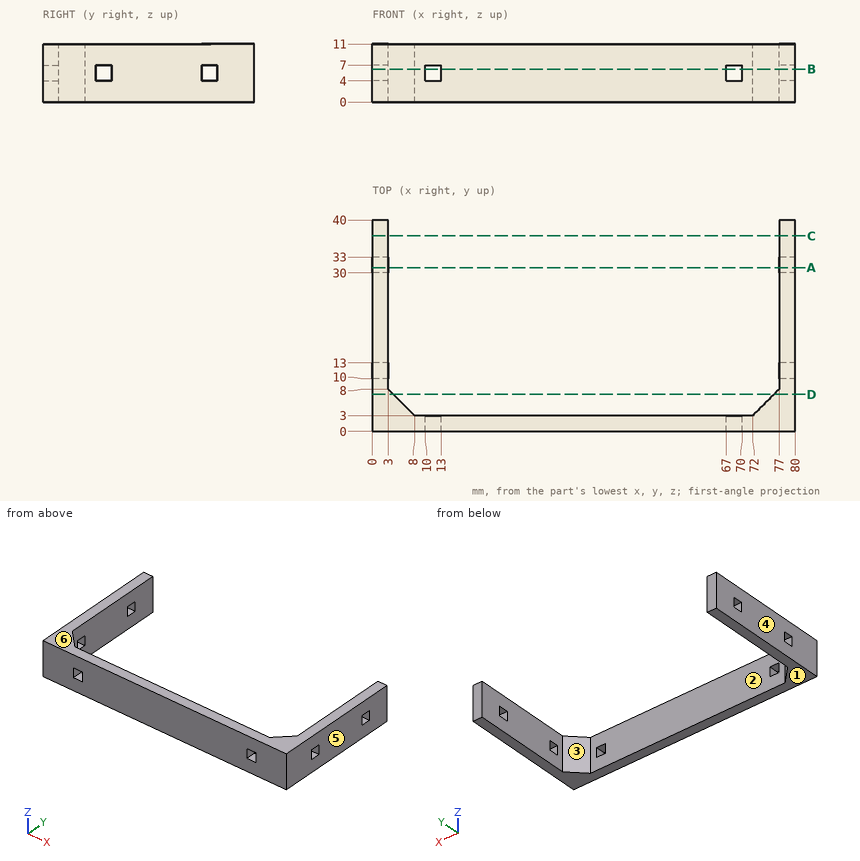
Job drawing, mm, ordinate dimensions from the low corner. One solid piece. A direction names the side the tool comes from. Coordinates: 2 decimals unless noted, no trailing zeros. Order: outer loops, then holes, each group sorted by start corner. A loop starts at its lowest first (then second) coordinate and runs counter-clockwise, first axis right, second up. Notation, with made-up numbers: (6, -3) - (10, -3) arc R36 ccw to (10, 33) - close; hole circle Ø5 at (66, 22.5). An arc over 180 degrees is marked (long way). Return JSON: item names as keys, results as strings. Group by question number.
1) Tool access for the marked faces 1 and 2: list every direction of +Z, -Z, +X, -X, +Y, -Y with a clear straight run to the whole face (end or side of a thin tool).
2) Probe line 1 (X direction, y = 2, z = 6.75); line 2 (X direction, y = 14, z = 9); line 3 (Y direction, x = 73, z = 9.75). List the from-to ranges inside material, lowest first. Write a range as from..to.
3) Mould opens along X. For the marked faces 3, 4, 5 and 6 say: released by +X, released by -X, zero draft, split by the parting line, or undercut.
4) Saw through at A-A, the plane y = 31. Write the cut outline in (x, z).
5) Saw through at C-C, the plane y = 37. Write the cut outline in (x, z), plus the area to 3 significant figures.
6) Saw through at D-D, the plane y = 7. Write the cut outline in (x, z).
7) Saw through at B-B, the plane z = 6.25. Count the separate pieces of the cut face and the enclosed holes in it, plus the area to 3 significant figures.
8) Flat gauge pin, fed straight in: P1, Ø2.5, axis at y = 1, z = 5, coming from the -X side. Where does the tip first touch, or does it go through?
Values found:
{
 "1": {"face 1": "-Z, +X, -X, +Y, -Y", "face 2": "+Z, -Z, +Y"},
 "2": {"line 1": "x = 0..10, 13..67, 70..80", "line 2": "x = 0..3, 77..80", "line 3": "y = 0..4"},
 "3": {"face 3": "undercut", "face 4": "released by -X", "face 5": "released by +X", "face 6": "zero draft"},
 "4": {"outline": "(0, 0) - (3, 0) - (3, 4) - (0, 4) - close; (0, 7) - (3, 7) - (3, 11) - (0, 11) - close; (77, 0) - (80, 0) - (80, 4) - (77, 4) - close; (77, 7) - (80, 7) - (80, 11) - (77, 11) - close"},
 "5": {"outline": "(0, 0) - (3, 0) - (3, 11) - (0, 11) - close; (77, 0) - (80, 0) - (80, 11) - (77, 11) - close", "area": "66.0 mm²"},
 "6": {"outline": "(0, 0) - (4, 0) - (4, 11) - (0, 11) - close; (76, 0) - (80, 0) - (80, 11) - (76, 11) - close"},
 "7": {"separate pieces": "7", "enclosed holes": "0", "area": "433 mm²"},
 "8": {"P1": "stops at x = 0"}
}
